```python
from build123d import *

# Parameters (mm, degrees)
BOSS_EXTRUDE1_DEPTH        = 7
F_9_0_9_DIAMETER_HOLE1_D   = 9
F_16_0_16_DIAMETER_HOLE1_D = 16
F_9_0_9_DIAMETER_HOLE2_D   = 9
CHAMFER1_SIZE              = 0.5
FILLET1_R                  = 3


with BuildPart() as part:
    # Sketch1 → Boss-Extrude1 (new body)
    with BuildSketch(Plane(origin=(0, 0, 0), x_dir=(-1, 0, 0), z_dir=(0, 0, -1))):
        Polygon((0, 0), (-100, 0), (-100, -20), (-20, -100), (0, -100), align=None)
    extrude(amount=-BOSS_EXTRUDE1_DEPTH)

    # Ø9.0 (9) Diameter Hole1 (through all)
    with Locations(Plane.XY.offset(7)):
        with Locations((85, -15), (15, -15)):
            Hole(F_9_0_9_DIAMETER_HOLE1_D / 2)

    # Ø16.0 (16) Diameter Hole1 (through all)
    with Locations(Plane.XY.offset(7)):
        with Locations((45, -45)):
            Hole(F_16_0_16_DIAMETER_HOLE1_D / 2)

    # Ø9.0 (9) Diameter Hole2 (through all)
    with Locations(Plane(origin=(0, 0, 0), x_dir=(-1, 0, 0), z_dir=(0, 0, -1))):
        with Locations((-15, -85)):
            Hole(F_9_0_9_DIAMETER_HOLE2_D / 2)

    # Chamfer1
    chamfer1_edges = [part.edges().sort_by_distance(p)[0] for p in [
        (19.5, -15, 7),
        (19.5, -15, 0),
        (89.5, -15, 7),
        (89.5, -15, 0),
        (53, -45, 7),
        (53, -45, 0),
        (10.5, -85, 0),
        (10.5, -85, 7),
    ]]
    chamfer(chamfer1_edges, length=CHAMFER1_SIZE)

    # Fillet1
    fillet1_edges = [part.edges().sort_by_distance(p)[0] for p in [
        (0, -100, 3.5),
        (20, -100, 3.5),
        (100, -20, 3.5),
        (100, 0, 3.5),
        (0, 0, 3.5),
    ]]
    fillet(fillet1_edges, radius=FILLET1_R)


solid = part.part
```
Part model, mm, in its own coordinate system. Round coordinates to 2 decimals unless told otherwise and drop trailing zeros. Loops run counter-clockwise (first coordinate to the right, second up) from the corner with the lowest first, then second, coordinate; pieces in that order, holes last. Notation, with made-up numbers: (40, 7.25) -> (99, 7.25) arc R34 ccw to (99, 40.25) -> close; hole circle Ø2 at (-30.75, 72.25). An arc over 180 degrees is marked (long way). Use a Markdown table: item, result.
1) Cut at C-C, the plane z = 2.75. List the corners of the cut face in (x, y), and give its area (3 significant figures).
The answers:
| item | result |
|---|---|
| outline | (0, -97) arc R3 ccw to (3, -100) -> (18.76, -100) arc R3 ccw to (20.88, -99.12) -> (99.12, -20.88) arc R3 ccw to (100, -18.76) -> (100, -3) arc R3 ccw to (97, 0) -> (3, 0) arc R3 ccw to (0, -3) -> close; hole circle Ø9 at (15, -85); hole circle Ø9 at (15, -15); hole circle Ø16 at (45, -45); hole circle Ø9 at (85, -15) |
| area | 6,400 mm2 |
2) Cut at B-B, the plane y = -45. List the corners of the cut face in (x, z).
The answers:
| item | result |
|---|---|
| outline | (0, 0) -> (36.5, 0) -> (37, 0.5) -> (37, 6.5) -> (36.5, 7) -> (0, 7) -> close; (53, 0.5) -> (53.5, 0) -> (75, 0) -> (75, 7) -> (53.5, 7) -> (53, 6.5) -> close |
3) Drop flat-ended pins along their axis: pin 1 Ø14.5 at (x, y) = (85, -15) entering from +Z; pin 2 Ø8 at (x, y) = (15, -15) entering from +Z; pin 3 Ø1.5 at (x, z) = (46, 3.5) entering from -Y; pin 4 Ø2 at (x, z) = (53.5, 2) entering from -Y. Give the stop position or say it passes through.
The answers:
| item | result |
|---|---|
| pin 1 | stops at z = 7 |
| pin 2 | passes through |
| pin 3 | stops at y = -74.75 |
| pin 4 | stops at y = -67.5 |
4) Cut at A-A, the plane x = 85. List the corners of the cut face in (y, z).
The answers:
| item | result |
|---|---|
| outline | (-35, 0) -> (-20, 0) -> (-19.5, 0.5) -> (-19.5, 6.5) -> (-20, 7) -> (-35, 7) -> close; (-10.5, 0.5) -> (-10, 0) -> (0, 0) -> (0, 7) -> (-10, 7) -> (-10.5, 6.5) -> close |
5) Cut at D-D, the plane y = -15. List the corners of the cut face in (x, z), and give its area (3 significant figures).
The answers:
| item | result |
|---|---|
| outline | (0, 0) -> (10, 0) -> (10.5, 0.5) -> (10.5, 6.5) -> (10, 7) -> (0, 7) -> close; (19.5, 0.5) -> (20, 0) -> (80, 0) -> (80.5, 0.5) -> (80.5, 6.5) -> (80, 7) -> (20, 7) -> (19.5, 6.5) -> close; (89.5, 0.5) -> (90, 0) -> (100, 0) -> (100, 7) -> (90, 7) -> (89.5, 6.5) -> close |
| area | 573 mm2 |
6) Pull direction Y, two halves, no side cores. Call faces 1 (the cylindrical face through (18.32, -11.96, 3.46)), 2 (the flat face through (11, -100, 3)), 3 (the flat face through (39.6, -38.2, 7)), 4 (the cylindrical face through (50.9, -39.6, 3.5)): pulls with the +Y half, pulls with the -Y half, needs draft (parallel to the pull), parting line crosses it, or undercut.
The answers:
| item | result |
|---|---|
| face 1 | undercut |
| face 2 | pulls with the -Y half |
| face 3 | needs draft |
| face 4 | undercut |
7) Probe line 1 (X direction, y = -14.5, z = 1.5); line 2 (Y direction, x = 15, z = 4.55); line 3 (Y direction, x = 18.5, z = 6). List the from-to ranges inside material, lowest first. Write a range as [from, to].
The answers:
| item | result |
|---|---|
| line 1 | x = [0, 10.53], [19.47, 80.53], [89.47, 100] |
| line 2 | y = [-100, -89.5], [-80.5, -19.5], [-10.5, 0] |
| line 3 | y = [-100, -87.83], [-82.17, -17.83], [-12.17, 0] |
